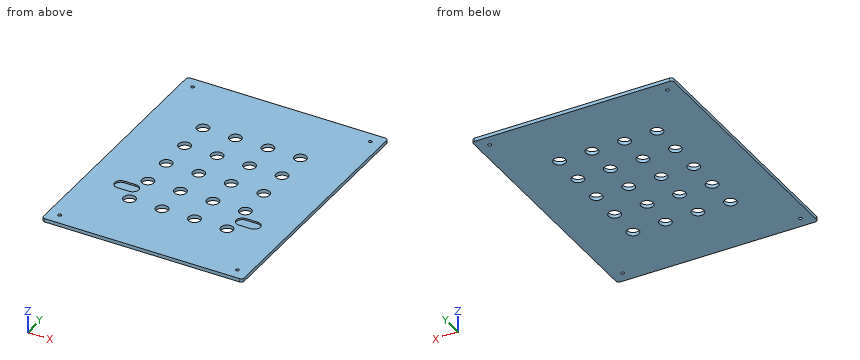
from build123d import *

# Parameters (mm, degrees)
F0_R     = 3
F1_DEPTH = 6
F2_R     = 10.5
F3_DEPTH = 25
F5_DEPTH = 3


with BuildPart() as f1:
    # F0 (on Top) → F1 (new body)
    with BuildSketch(Plane.XY):
        with BuildLine():
            Line((170, 225), (-170, 225))
            ThreePointArc((-170, 225), (-173.535534, 223.535534), (-175, 220))
            Line((-175, 220), (-175, -220))
            ThreePointArc((-175, -220), (-173.535534, -223.535534), (-170, -225))
            Line((-170, -225), (170, -225))
            ThreePointArc((170, -225), (173.535534, -223.535534), (175, -220))
            Line((175, -220), (175, 220))
            ThreePointArc((175, 220), (173.535534, 223.535534), (170, 225))
        make_face()
        with Locations((-155, -205.25)):
            Circle(F0_R, mode=Mode.SUBTRACT)
        with Locations((155, -205.25)):
            Circle(F0_R, mode=Mode.SUBTRACT)
        with Locations((-155, 205.25)):
            Circle(F0_R, mode=Mode.SUBTRACT)
        with Locations((155, 205.25)):
            Circle(F0_R, mode=Mode.SUBTRACT)
    extrude(amount=F1_DEPTH)

    # F2 (on face) → F3 (cut)
    with BuildSketch(Plane.XY.offset(6)):
        with Locations((-85, 113.333333)):
            Circle(F2_R)
        with Locations((-85, 56.666667)):
            Circle(F2_R)
        with Locations((-85, 0)):
            Circle(F2_R)
        with Locations((-85, -56.666667)):
            Circle(F2_R)
        with Locations((-85, -113.333333)):
            Circle(F2_R)
        with Locations((-28.333333, -113.333333)):
            Circle(F2_R)
        with Locations((-28.333333, -56.666667)):
            Circle(F2_R)
        with Locations((-28.333333, 0)):
            Circle(F2_R)
        with Locations((-28.333333, 56.666667)):
            Circle(F2_R)
        with Locations((-28.333333, 113.333333)):
            Circle(F2_R)
        with Locations((28.333333, 113.333333)):
            Circle(F2_R)
        with Locations((28.333333, 56.666667)):
            Circle(F2_R)
        with Locations((28.333333, 0)):
            Circle(F2_R)
        with Locations((28.333333, -56.666667)):
            Circle(F2_R)
        with Locations((28.333333, -113.333333)):
            Circle(F2_R)
        with Locations((85, -113.333333)):
            Circle(F2_R)
        with Locations((85, -56.666667)):
            Circle(F2_R)
        with Locations((85, 0)):
            Circle(F2_R)
        with Locations((85, 56.666667)):
            Circle(F2_R)
        with Locations((85, 113.333333)):
            Circle(F2_R)
    extrude(amount=-F3_DEPTH, mode=Mode.SUBTRACT)

    # F4 (on face) → F5 (cut)
    with BuildSketch(Plane.XY.offset(6)):
        with BuildLine():
            Line((-95.5, -74.5), (-116.5, -74.5))
            ThreePointArc((-116.5, -74.5), (-127, -85), (-116.5, -95.5))
            Line((-116.5, -95.5), (-95.5, -95.5))
            ThreePointArc((-95.5, -95.5), (-85, -85), (-95.5, -74.5))
        make_face()
        with BuildLine():
            ThreePointArc((116.5, -95.5), (127, -85), (116.5, -74.5))
            Line((116.5, -74.5), (95.5, -74.5))
            ThreePointArc((95.5, -74.5), (85, -85), (95.5, -95.5))
            Line((95.5, -95.5), (116.5, -95.5))
        make_face()
    extrude(amount=-F5_DEPTH, mode=Mode.SUBTRACT)


solid = f1.part
Geometry check sheet. Reference: the model listing, model coordinates, mm. Give positions to 0.01 mm unless a question says otherwise; leave off trailing zeros. Loops run counter-clockwise (first coordinate to the right, second up) from the corner with the lowest first, then second, coordinate; pieces in that order, holes last. Notation, with made-up numbers: M 87.5,82.5 L 123.5,82.5 A30 ccw 123.5,114.5 Z; hole C 0,67.5 d3. An arc over 180 degrees is marked long. Answer as a JSON object with one key per item and string values. Group by question number.
Item 1: Gauge pin test, flat end, axial feed: pin 1 (6.5 mm diameter, centred on x = -99.5, y = -81, fed in from +Z). Record the tip position at first contact, or that the pin passes through.
Item 2: Sectioned sample at A-A on y = 0. Record the boundary of the cut face in (x, z), plus the area to 3 significant figures.
Item 3: Material ranges on L1, parallel to X at y = 119, z = 1.35; L2, parallel to X at y = 206, z = 5.4; L3, parallel to Y at x = -30, z = 3.1, recorded low to high.
Item 4: Sectioned sample at B-B on z = 1.05. Give the number of separate pieces and of enclosed holes in the cut face, plus the area to 3 significant figures.
Item 5: Sectioned sample at D-D on x = 33.5. Record the boundary of the cut face in (y, z), plus the area to 3 significant figures.
Item 6: Sectioned sample at C-C on x = -110. Record the boundary of the cut face in (y, z).
Findings below:
{
 "1": {"pin 1": "z = 3"},
 "2": {"outline": "M -175,0 L -95.5,0 L -95.5,6 L -175,6 Z; M -74.5,0 L -38.83,0 L -38.83,6 L -74.5,6 Z; M -17.83,0 L 17.83,0 L 17.83,6 L -17.83,6 Z; M 38.83,0 L 74.5,0 L 74.5,6 L 38.83,6 Z; M 95.5,0 L 175,0 L 175,6 L 95.5,6 Z", "area": "1,600 mm2"},
 "3": {"L1": "-175 to -93.84, -76.16 to -37.17, -19.49 to 19.49, 37.17 to 76.16, 93.84 to 175", "L2": "-175 to -157.9, -152.1 to 152.1, 157.9 to 175", "L3": "-225 to -123.7, -102.97 to -67.03, -46.3 to -10.37, 10.37 to 46.3, 67.03 to 102.97, 123.7 to 225"},
 "4": {"separate pieces": "1", "enclosed holes": "24", "area": "150,000 mm2"},
 "5": {"outline": "M -225,0 L -122.47,0 L -122.47,6 L -225,6 Z; M -104.19,0 L -65.81,0 L -65.81,6 L -104.19,6 Z; M -47.53,0 L -9.14,0 L -9.14,6 L -47.53,6 Z; M 9.14,0 L 47.53,0 L 47.53,6 L 9.14,6 Z; M 65.81,0 L 104.19,0 L 104.19,6 L 65.81,6 Z; M 122.47,0 L 225,0 L 225,6 L 122.47,6 Z", "area": "2,150 mm2"},
 "6": {"outline": "M -225,0 L 225,0 L 225,6 L -74.5,6 L -74.5,3 L -95.5,3 L -95.5,6 L -225,6 Z"}
}
